Verification items for this drawing (mm, ordinates from the low corner). Give positions to 0.01 mm unless a question says otherwise; leave off trailing zeros. Loops run counter-clockwise (first coordinate to the right, second up) from the corner with the lowest first, then second, coordinate; pieces in that order, holes last. Notation, with made-up numbers: (-25, 10) -> (-3, 10) arc R35 cw to (-3, 47) -> close; hole circle Ø3 at (13, 70). An arc over 180 degrees is marked (long way). Write item = value, one per line.
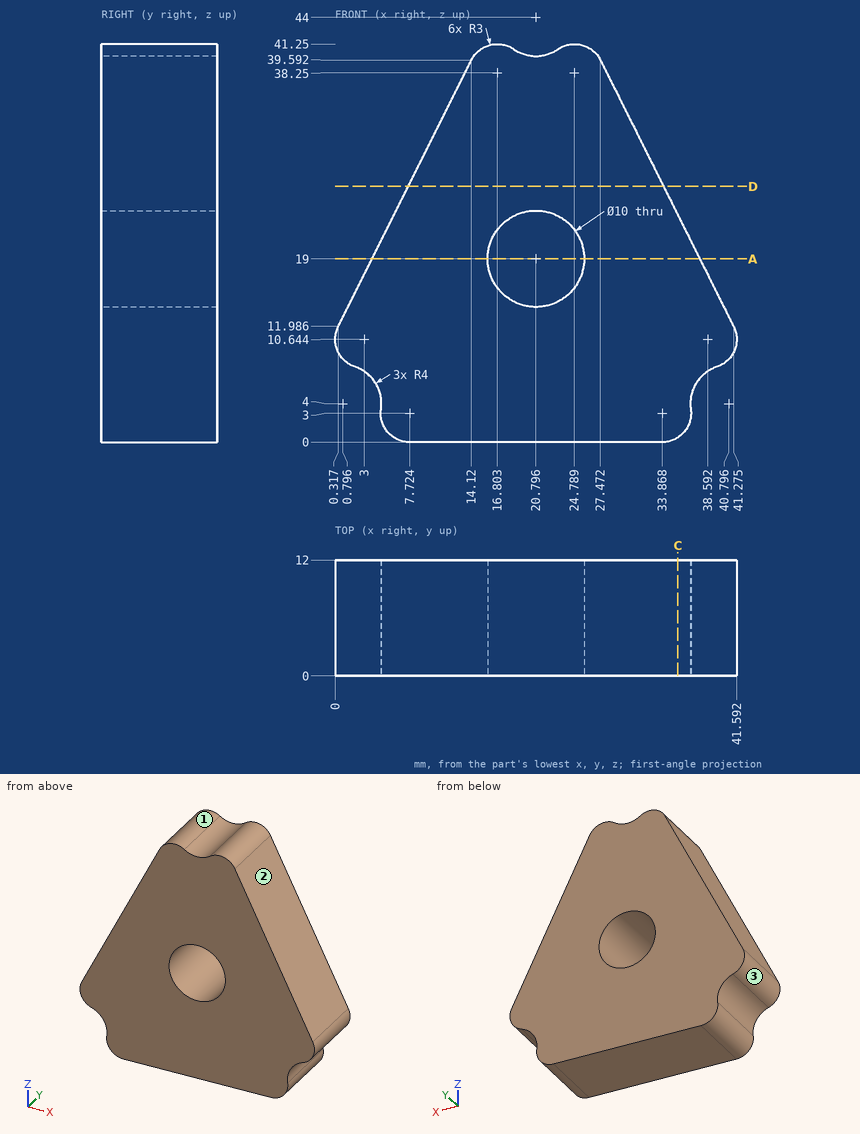
Item 1: Gauge pin test, flat ends, axial feed: pin 1 (6 mm diameter, centred on x = 20.8, z = 19, fed in from -Y); pin 2 (1 mm diameter, centred on x = 34.5, y = 3, fed in from -Z); pin 3 (5 mm diameter, centred on y = 4, z = 19, fed in from +X). Record the tip position at first contact, or that the pin passes through.
Answer:
pin_1 = through
pin_2 = 0
pin_3 = 39.02
Item 2: Draft check along X on the marked faces 1, 2 and 3. Enter one of: +X half, -X half, draft (parallel to the pull), parting line (faces both ways), or undercut.
Answer:
face_1 = undercut
face_2 = +X half
face_3 = -X half
Item 3: Section check C-C, the plane x = 35.5. Record the cut outline in (y, z), plus the area to 3 significant figures.
Answer:
outline = (0, 0.48) -> (12, 0.48) -> (12, 23.54) -> (0, 23.54) -> close
area = 277 mm^2
Item 4: Thickness scan on L1, parallel to Z at x = 21, y = 9.75 (1 decimal); L2, parallel to X at y = 2.5, z = 15.5 (1 decimal); L3, parallel to X at y = 4.5, z = 19 (1 decimal). Record the ranges inside material, lowest first. Write a range as [from, to].
Answer:
L1 = [0, 14], [24, 40]
L2 = [2.1, 17.2], [24.4, 39.5]
L3 = [3.8, 15.8], [25.8, 37.8]
Item 5: Section check D-D, the plane z = 26.5. Record the cut outline in (x, y), plus the area to 3 significant figures.
Answer:
outline = (7.57, 0) -> (34.02, 0) -> (34.02, 12) -> (7.57, 12) -> close
area = 317 mm^2
Item 6: Section check A-A, the plane z = 19. Record the cut outline in (x, y).
Answer:
outline = (3.82, 0) -> (15.8, 0) -> (15.8, 12) -> (3.82, 12) -> close; (25.8, 0) -> (37.77, 0) -> (37.77, 12) -> (25.8, 12) -> close
